Source: CAD feature listing. Evaluate the final solid. Frame: model axes, mm. A direction names the side the tool comes from. Round coordinates to 2 decimals unless told otherwise and drop trailing zeros. Order: outer loops, then holes, each group sorted by start corner. A loop starts at its lowest first (then second) coordinate and runs counter-clockwise, first axis right, second up. Notation, with made-up numbers: (4.25, 33) - (28.25, 33) arc R21 cw to (28.25, 41) - close; hole circle Ø8 at (-6.75, -21). An arc over 180 degrees is marked (long way). Put each result on its own line as item: value. Start each with the question number.
1) Section A-A on x = 17.5. Output: boundary loops of the cut face in (y, z), then the cut area to 4 significant figures.
2) Access query for faces 1 (the face through (-1, 1, 0)), 2 (the face through (-1, 0, 1.5)). Directions: +Z, -Z, +X, -X, +Y, -Y. A direction counts if a zero-diameter tool reaches every point of the face in a straight line with its end or side. Return the directions, or none.
3) Line query: probe 1 along Z at (x, y) = (55, 17.5); probe 2 along Y at (x, z) = (-3, 13.25). Output: solid intervals per line, ascending. Write a range as [from, to].
4) Section D-D on z = 11. Output: boundary loops of the cut face in (x, y), then the cut area to 3 significant figures.
5) Section B-B on y = 18. Output: boundary loops of the cut face in (x, z), then the cut area to 3 significant figures.
6) Contact query for flat-ended pins moving along their axis: P1, Ø6, axis at x = -15.5, y = 52, coming from the -Z side; P2, Ø12, axis at x = 6.5, y = -50.5, coming from the +Z side. Output: stop coordinate, or through.
7) Section C-C on x = -43.5. Output: boundary loops of the cut face in (y, z), then the cut area to 4 significant figures.
```python
from build123d import *

# Parameters (mm, degrees)
F2_W     = 130
F2_H     = 140.5
F3_DEPTH = 1.5
F2_H_2   = 1.5
F4_DEPTH = 16.5
F5_W     = 80
F5_H     = 2
F6_DEPTH = 1.501


with BuildPart() as f3:
    # F2 (on Top) → F3 (new body)
    with BuildSketch(Plane.XY):
        with Locations((0, -0.75)):
            Rectangle(F2_W, F2_H)
    extrude(amount=F3_DEPTH)

    # F2 (on Top) → F4 (join)
    with BuildSketch(Plane.XY):
        with Locations((0, 70.25)):
            Rectangle(F2_W, F2_H_2)
    extrude(amount=F4_DEPTH)

    # F5 (on face) → F6 (cut, through all)
    with BuildSketch(Plane.XY.offset(1.5)):
        with Locations((0, 28.5)):
            Rectangle(F5_W, F5_H)
        with Locations((0, 3.5)):
            Rectangle(F5_W, F5_H)
        with Locations((0, -21.5)):
            Rectangle(F5_W, F5_H)
    extrude(amount=-F6_DEPTH, mode=Mode.SUBTRACT)


solid = f3.part
```
Answer sheet:
1. outline: (-71, 0) - (-22.5, 0) - (-22.5, 1.5) - (-71, 1.5) - close; (-20.5, 0) - (2.5, 0) - (2.5, 1.5) - (-20.5, 1.5) - close; (4.5, 0) - (27.5, 0) - (27.5, 1.5) - (4.5, 1.5) - close; (29.5, 0) - (71, 0) - (71, 16.5) - (69.5, 16.5) - (69.5, 1.5) - (29.5, 1.5) - close
1. area: 226.5 mm^2
2. face 1: -Z, +X, -X, +Y, -Y
2. face 2: +Z, +X, -X, -Y
3. probe 1: [0, 1.5]
3. probe 2: [69.5, 71]
4. outline: (-65, 69.5) - (65, 69.5) - (65, 71) - (-65, 71) - close
4. area: 195 mm^2
5. outline: (-65, 0) - (65, 0) - (65, 1.5) - (-65, 1.5) - close
5. area: 195 mm^2
6. P1: z = 0
6. P2: z = 1.5
7. outline: (-71, 0) - (71, 0) - (71, 16.5) - (69.5, 16.5) - (69.5, 1.5) - (-71, 1.5) - close
7. area: 235.5 mm^2
